Design review of the part built by this model. Coordinates are the model's own, in mm. Face numbers are marked on the shaded views. A direction names the side the tool comes from. Coordinates: 2 decimals unless noted, no trailing zeros. Order: outer loops, then holes, each group sorted by start corner. A loop starts at its lowest first (then second) coordinate and runs counter-clockwise, first axis right, second up. Notation, with made-up numbers: (75, -29) -> (80, -29) arc R10 cw to (80, -15) -> close; hole circle Ø8 at (79.5, 62). An arc over 180 degrees is marked (long way). Use a Markdown table: item, result. Add a question column.
Q1. Add section B-B (y = -60.5). State the section outline as (x, z) points.
Q2. Wall thickness on probe 1 along X at (y, z) = (92, -789); probe 2 along X at (y, z) = (82, -787.4); probe 3 along Y at (x, z) = (196, -477): over which ranges is each line inside the solid? List them lowest first.
Q3. Add section A-A (x = -77.5). State the section outline as (y, z) points.
Q4. Insertion check: pin 1 (4 mm diameter, centred on x = -124, z = -786, fed in from -Y); pin 2 (14 mm diameter, centred on x = 126.5, z = -786.5, fed in from -Y); pin 3 (4 mm diameter, centred on y = 79, z = -621, fed in from +X). Each pin has a flat end and moves straight along its axis. Give the tip position at first contact, or say it passes through.
Q5. Machinability: for the marked faces 1 and 2, which of the approach directions +Z, -Z, +X, -X, +Y, -Y give a long, thin tool a straight path to every point of the face, cutting with its end or side? Answer none if there is none.
Q6. Add section C-C (z = -125). State the section outline as (x, y) points, then the cut area to 3 significant figures.
from build123d import *

# Parameters (mm, degrees)
SKETCH1_R           = 12.7
BOSS_EXTRUDE1_DEPTH = 254
FILLET1_R           = 8.382
FILLET2_R           = 8.382
SKETCH6_W           = 445.900168358
SKETCH6_H           = 171.500064753
CUT_EXTRUDE4_DEPTH  = 1009.8530191
SKETCH2_R           = 6.35
CUT_EXTRUDE5_DEPTH  = 38.1


with BuildPart() as part:
    # Sketch1 → Boss-Extrude1 (new, symmetric)
    with BuildSketch(Plane(origin=(0, 0, 0), x_dir=(0, 0, -1), z_dir=(1, 0, 0))):
        Polygon((-50.8, 122.075554067), (914.4, 122.075554067), (914.4, 72.291554067), (0, 72.291554067), (0, -147.164445933), (-50.8, -147.164445933), align=None)
        with Locations((-25.220095835, -101.724479604)):
            Circle(SKETCH1_R, mode=Mode.SUBTRACT)
    extrude(amount=BOSS_EXTRUDE1_DEPTH, both=True)

    # Fillet1
    fillet1_edges = [part.edges().sort_by_distance(p)[0] for p in [
        (0, 122.075554067, 50.8),
        (0, 122.075554067, -914.4),
        (0, 72.291554067, -914.4),
        (0, -147.164445933, 50.8),
        (254, -37.436445933, 0),
        (254, 72.291554067, -457.2),
        (254, 97.183554067, -914.4),
        (254, 122.075554067, -431.8),
        (254, -12.544445933, 50.8),
        (-254, 122.075554067, -431.8),
        (-254, 97.183554067, -914.4),
        (-254, -12.544445933, 50.8),
    ]]
    fillet(fillet1_edges, radius=FILLET1_R)

    # Fillet2
    # the kernel refuses this fillet: 8.382 mm, written as the material it takes off along each edge
    with BuildSketch(Plane(origin=(245.618, -138.782445933, 42.418), x_dir=(0, -1, 0), z_dir=(1, 0, 0))) as fillet2_piece_1_section:
        Polygon((0, 0), (FILLET2_R, 0), (FILLET2_R, -FILLET2_R), (0, -FILLET2_R), align=None)
    fillet2_piece_1 = extrude(amount=FILLET2_R, mode=Mode.PRIVATE)
    fillet2_piece_1 = fillet2_piece_1 - Plane(origin=(245.618, -138.782445933, 42.418), x_dir=(0, 0.7071067811865477, -0.7071067811865474), z_dir=(1, 0, 0)) * Sphere(FILLET2_R, mode=Mode.PRIVATE)
    add(fillet2_piece_1, mode=Mode.SUBTRACT)
    with BuildSketch(Plane(origin=(-245.618, -138.782445933, 42.418), x_dir=(0, -1, 0), z_dir=(-1, 0, 0))) as fillet2_piece_2_section:
        Polygon((0, 0), (FILLET2_R, 0), (FILLET2_R, FILLET2_R), (0, FILLET2_R), align=None)
    fillet2_piece_2 = extrude(amount=FILLET2_R, mode=Mode.PRIVATE)
    fillet2_piece_2 = fillet2_piece_2 - Plane(origin=(-245.618, -138.782445933, 42.418), x_dir=(0, 0.7071067811865477, -0.7071067811865474), z_dir=(-1, 0, 0)) * Sphere(FILLET2_R, mode=Mode.PRIVATE)
    add(fillet2_piece_2, mode=Mode.SUBTRACT)
    with BuildSketch(Plane(origin=(254, -147.164445933, 8.382), x_dir=(0, 1, 0), z_dir=(0, 0, 1))) as fillet2_piece_3:
        with BuildLine():
            CenterArc((FILLET2_R, FILLET2_R), FILLET2_R, 180, 90)
            Line((0, FILLET2_R), (0, 0))
            Line((0, 0), (FILLET2_R, 0))
        make_face()
    extrude(amount=34.036, mode=Mode.SUBTRACT)
    with BuildSketch(Plane(origin=(-254, -147.164445933, -20.955), x_dir=(0, 1, 0), z_dir=(0, 0, 1))) as fillet2_piece_4:
        with BuildLine():
            CenterArc((FILLET2_R, -FILLET2_R), FILLET2_R, 90, 90)
            Line((0, -FILLET2_R), (0, 0))
            Line((0, 0), (FILLET2_R, 0))
        make_face()
    extrude(amount=63.373, mode=Mode.SUBTRACT)
    with BuildSketch(Plane(origin=(-274.955, -147.164445933, 0), x_dir=(0, 1, 0), z_dir=(1, 0, 0))) as fillet2_piece_5:
        with BuildLine():
            CenterArc((FILLET2_R, FILLET2_R), FILLET2_R, 180, 90)
            Line((0, FILLET2_R), (0, 0))
            Line((0, 0), (FILLET2_R, 0))
        make_face()
    extrude(amount=520.573, mode=Mode.SUBTRACT)
    with BuildSketch(Plane(origin=(245.618, -147.164445933, 8.382), x_dir=(1, 0, 0), z_dir=(0, 0, 1))) as fillet2_piece_6:
        with BuildLine():
            CenterArc((8.382 - FILLET2_R, FILLET2_R), FILLET2_R, 270, 90)
            Line((8.382, FILLET2_R), (8.382, 0))
            Line((8.382, 0), (8.382 - FILLET2_R, 0))
        make_face()
    revolve(axis=Axis((245.618, -147.164445933, 8.382), (0, 1, 0)), revolution_arc=90, mode=Mode.SUBTRACT)

    # Sketch6 → Cut-Extrude4 (cut, through all)
    with BuildSketch(Plane.XY.offset(50.8)):
        with Locations((-3.610527679, -37.818139686)):
            Rectangle(SKETCH6_W, SKETCH6_H)
    extrude(amount=-CUT_EXTRUDE4_DEPTH, mode=Mode.SUBTRACT)

    # Sketch2 → Cut-Extrude5 (cut)
    with BuildSketch(Plane.XZ.offset(-72.291554067)):
        with Locations(Location((-127, -787.4, 0), (0, 0, 270))):
            Circle(SKETCH2_R)
        with Locations(Location((127, -787.4, 0), (0, 0, 270))):
            Circle(SKETCH2_R)
    extrude(amount=-CUT_EXTRUDE5_DEPTH, mode=Mode.SUBTRACT)


solid = part.part
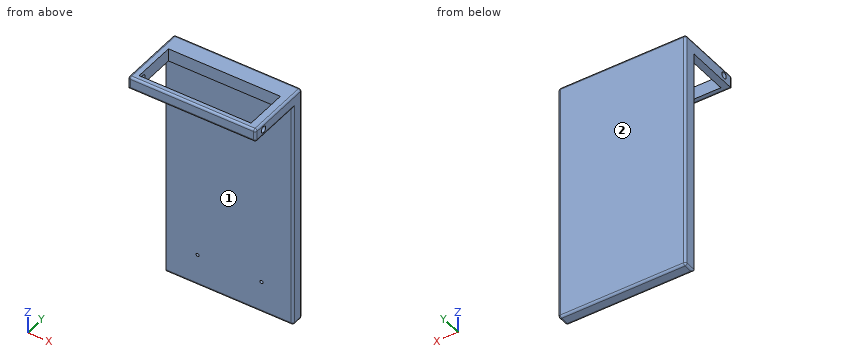
Established:
| question | item | result |
|---|---|---|
| 1 | outline | (-254, 0) -> (-226.56, 0) -> (-226.56, 50.8) -> (-245.62, 50.8) arc R8.38 ccw to (-254, 42.42) -> close; (219.34, 0) -> (245.62, 0) arc R8.38 ccw to (254, 8.38) -> (254, 42.42) arc R8.38 ccw to (245.62, 50.8) -> (219.34, 50.8) -> close |
| 2 | probe 1 | -254 to -133.15, -120.85 to 120.85, 133.15 to 254 |
| 2 | probe 2 | -254 to -133.35, -120.65 to 120.65, 133.35 to 254 |
| 2 | probe 3 | 72.29 to 122.08 |
| 3 | outline | (-147.16, 8.38) arc R8.38 ccw to (-138.78, 0) -> (-123.57, 0) -> (-123.57, 50.8) -> (-138.78, 50.8) arc R8.38 ccw to (-147.16, 42.42) -> close; (47.93, 0) -> (72.29, 0) -> (72.29, -906.02) arc R8.38 ccw to (80.67, -914.4) -> (113.69, -914.4) arc R8.38 ccw to (122.08, -906.02) -> (122.08, 42.42) arc R8.38 ccw to (113.69, 50.8) -> (47.93, 50.8) -> close |
| 4 | pin 1 | y = 110.39 |
| 4 | pin 2 | y = 72.29 |
| 4 | pin 3 | x = 254 |
| 5 | face 1 | -Z, +X, -X, -Y |
| 5 | face 2 | +Z, -Z, +X, -X, +Y |
| 6 | outline | (-254, 72.29) -> (245.62, 72.29) arc R8.38 ccw to (254, 80.67) -> (254, 113.69) arc R8.38 ccw to (245.62, 122.08) -> (-245.62, 122.08) arc R8.38 ccw to (-254, 113.69) -> close |
| 6 | area | 25,200 mm^2 |
